```python
from build123d import *

# Parameters (mm, degrees)
F0_R     = 2.4257
F1_DEPTH = 2.54


with BuildPart() as f1:
    # F0 (on Top) → F1 (new body)
    with BuildSketch(Plane.XY):
        with BuildLine():
            ThreePointArc((10.31875, 7.403607), (0, -12.7), (-10.31875, 7.403607))
            Line((-10.31875, 7.403607), (-10.31875, 8.995426))
            ThreePointArc((-10.31875, 8.995426), (-10.947542, 9.624218), (-10.31875, 10.25301))
            Line((-10.31875, 10.25301), (-10.31875, 18.983854))
            ThreePointArc((-10.31875, 18.983854), (-12.178622, 23.473982), (-16.66875, 25.333854))
            Line((-16.66875, 25.333854), (-51.678968, 25.333854))
            ThreePointArc((-51.678968, 25.333854), (-52.440968, 25.079854), (-52.898168, 24.419454))
            Line((-52.898168, 24.419454), (-53.536901, 22.229512))
            Line((-53.536901, 22.229512), (-65.277999, 25.653999))
            ThreePointArc((-65.277999, 25.653999), (-67.114483, 26.529079), (-68.58, 27.94))
            ThreePointArc((-68.58, 27.94), (-83.100222, 28.791015), (-81.529968, 14.330884))
            Line((-81.529968, 14.330884), (-24.332909, -27.222641))
            ThreePointArc((-24.332909, -27.222641), (-0.623226, -36.507181), (23.389548, -28.037327))
            Line((23.389548, -28.037327), (80.234168, 13.596494))
            Line((80.234168, 13.596494), (83.209212, 15.775459))
            ThreePointArc((83.209212, 15.775459), (82.289932, 29.548821), (68.58, 27.94))
            ThreePointArc((68.58, 27.94), (67.114483, 26.529079), (65.277999, 25.653999))
            Line((65.277999, 25.653999), (53.540294, 22.230502))
            Line((53.540294, 22.230502), (52.90185, 24.419454))
            ThreePointArc((52.90185, 24.419454), (52.44465, 25.079854), (51.68265, 25.333854))
            Line((51.68265, 25.333854), (16.66875, 25.333854))
            ThreePointArc((16.66875, 25.333854), (12.178622, 23.473982), (10.31875, 18.983854))
            Line((10.31875, 18.983854), (10.31875, 10.259218))
            ThreePointArc((10.31875, 10.259218), (10.95375, 9.624218), (10.31875, 8.989218))
            Line((10.31875, 8.989218), (10.31875, 7.403607))
        make_face()
        with Locations((-76.2, 22.225)):
            Circle(F0_R, mode=Mode.SUBTRACT)
        with Locations((76.2, 22.225)):
            Circle(F0_R, mode=Mode.SUBTRACT)
        with BuildLine():
            ThreePointArc((80.234168, 13.596494), (81.828146, 14.540627), (83.209212, 15.775459))
            Line((83.209212, 15.775459), (80.234168, 13.596494))
        make_face()
    extrude(amount=F1_DEPTH)


solid = f1.part
```
The listing builds one solid part. Answer for the finished solid, in the listing's coordinates (mm). A direction names the side the tool comes from. Coordinates: 2 decimals unless noted, no trailing zeros. Loops run counter-clockwise (first coordinate to the right, second up) from the corner with the lowest first, then second, coordinate; pieces in that order, holes last. Notation, with made-up numbers: M -8.5,-30 L 0.5,-30 A15 ccw 0.5,-2 Z; hole C 84.25,-35.75 d6. An arc over 180 degrees is marked long. Answer as a JSON object with one key per item and string values. Group by question number.
Item 1: Section C-C (x = -76.2) is taken. Write down the section's boundary in (y, z).
Item 2: Each of these flat-tipped pins is pushed along its axis until it touches: P1, Ø6.5, axis at x = 76.2, y = 22.225, coming from the -Z side; P2, Ø1.3, axis at x = 35, z = 1.5, coming from the +Y side; P3, Ø0.8, axis at y = 8, z = 1, coming from the +X side. Where does it stop, or does it pass through?
Item 3: Which of the six approach directions +Z, -Z, +X, -X, +Y, -Y give full straight-line access (tool end or side, diameter ignored) to faces 1 (the face through (0.39, -12.694, 1.252)), 2 (the face through (12.228, 23.523, 1.252))?
Item 4: Section D-D (x = 0) is taken. Write down the section's boundary in (y, z), and give its area (3 significant figures).
Item 5: Consider L1, parallel to X at y = 20, z = 2.4; L2, parallel to Y at x = 0, z = 1.2; L3, parallel to Y at x = 76.2, z = 1.85. Determine where each line is inside the solid, lowest interval first.
Item 6: Section B-B (z = 2) is taken. Give the number of separate pieces and of enclosed holes in the cut face, and give its area (3 significant figures).
Item 7: Section A-A (y = 12) is taken. Write down the section's boundary in (x, z), and give its area (3 significant figures).
Item 8: Determine the mould class of faces 3 (the face through (51.414, -7.512, 1.252)), 4 (the face through (82.455, 29.409, 1.252)), 5 (the face through (18, 6, 2.54)) for opening direction X: +X half, -X half, draft (parallel to the pull), parting line (faces both ways), or undercut.
Solved:
{
 "1": {"outline": "M 10.46,0 L 19.8,0 L 19.8,2.54 L 10.46,2.54 Z; M 24.65,0 L 31.75,0 L 31.75,2.54 L 24.65,2.54 Z"},
 "2": {"P1": "stops at z = 0", "P2": "stops at y = 25.33", "P3": "stops at x = 73.14"},
 "3": {"face 1": "+Z, -Z", "face 2": "+Z, -Z, +Y"},
 "4": {"outline": "M -36.51,0 L -12.7,0 L -12.7,2.54 L -36.51,2.54 Z", "area": "60.5 mm2"},
 "5": {"L1": "x = -85.46 to -77.17, -75.23 to -10.4, 10.4 to 75.23, 77.17 to 85.46", "L2": "y = -36.51 to -12.7", "L3": "y = 10.64 to 19.8, 24.65 to 31.75"},
 "6": {"separate pieces": "1", "enclosed holes": "2", "area": "5,850 mm2"},
 "7": {"outline": "M -78.32,0 L -10.32,0 L -10.32,2.54 L -78.32,2.54 Z; M 10.32,0 L 78.05,0 L 78.05,2.54 L 10.32,2.54 Z", "area": "345 mm2"},
 "8": {"face 3": "+X half", "face 4": "undercut", "face 5": "draft"}
}
